CAD build for the part. Positions are in the model's coordinates, mm. A direction names the side the tool comes from. Coordinates: 2 decimals unless noted, no trailing zeros.
1) Wall check: line 1 along X through (y, z) = (-19, 4.5); line 2 along X through (y, z) = (-25.5, 2); line 3 along Y through (x, z) = (-2, 4.5). Give the ranges that are in metal, low to high.
2) Pin check, flat tips, straight feed: pin 1 Ø6 at (x, y) = (31.5, 18.5) entering from -Z; pin 2 Ø1.5 at (y, z) = (9.5, 3.5) entering from +X; pin 3 Ø6.5 at (y, z) = (-28, 5.5) entering from -X; pin 4 Ø5 at (y, z) = (15.5, 0.5) entering from +X. Stop position of each tip, or through.
3) Two-plate mould, pull along Y, no slides. Class faces 1 (the flat face through (13, -13, 0)), 2 (the cylindrical face through (-7, 6, 0)), 3 (the flat face through (22.815, 2.59, 2.465)), 4 (the flat face through (25, -50, 6)): +Y half, -Y half, draft (parallel to the pull), parting line (faces both ways), or undercut.
4) Which spindle directions (+Z, -Z, +X, -X, +Y, -Y) get a long thin tool onto all of the face, cutting with end or side? Do faces 5 (the flat face through (45, -22, 8)), 6 (the cylindrical face through (48, -22, 12)), 7 (the flat face through (-22, 0, -1)), 8 (the flat face through (22.81, -15.74, 2.46)), 9 (the flat face through (6, -6, 5)). Say none if no direction does.
5) Saw through at A-A, the plane y = -23. Give the number of separate pieces and of enclosed holes in the cut face, and give its area (3 significant figures).
```python
from build123d import *

# Parameters (mm, degrees)
F1_DEPTH  = 5
F3_DEPTH  = 5
F5_DEPTH  = 8
F6_SIZE   = 4.99999
F7_R      = 4.99999
F9_DEPTH  = 5
F11_DEPTH = 5


# Not quite as in the source:
# - a fillet or chamfer is up to 0.001 mm smaller than in the source, because OpenCascade refuses the exact size


with BuildPart() as f1:
    # F0 (on Top) → F1 (new body)
    with BuildSketch(Plane.XY):
        Polygon((0, 45), (-5, 45), (-5, 5), (-45, 5), (-45, 0), (0, -45), (0, -50), (50, -50), (50, 0), (45, 0), align=None)
        Polygon((45, -7.0710678119), (45, -45), (7.0710678119, -45), (-37.9289321881, 0), (0, 0), (0, 37.9289321881), align=None, mode=Mode.SUBTRACT)
    extrude(amount=F1_DEPTH)

    # F2 (on face) → F3 (join)
    with BuildSketch(Plane(origin=(0, 0, 0), x_dir=(1, 0, 0), z_dir=(0, 0, -1))):
        Polygon((0, -45), (0, 0), (-45, 0), (-45, -5), (-5, -5), (-5, -45), align=None)
    extrude(amount=F3_DEPTH)

    # F4 (on face) → F5 (join)
    with BuildSketch(Plane.XY.offset(5)):
        Polygon((50, 0), (45, 0), (45, -45), (0, -45), (0, -50), (50, -50), align=None)
    extrude(amount=F5_DEPTH)

    # F6 (size 5 in the source; OpenCascade refuses exactly that, so slightly less here)
    f6_edges = [f1.edges().sort_by_distance(p)[0] for p in [
        (0, -50, 6.5),
        (50, 0, 6.5),
    ]]
    chamfer(f6_edges, length=F6_SIZE)

    # F7 (radius 5 in the source; OpenCascade refuses exactly that, so slightly less here)
    f7_edges = [f1.edges().sort_by_distance(p)[0] for p in [
        (50, -50, 6.5),
        (-5, 45, 0),
        (-45, 5, 0),
        (-5, 5, 0),
        (50, -27.499995, 13),
        (27.499995, -50, 13),
        (27.499995, -50, 0),
        (50, -27.499995, 0),
    ]]
    fillet(f7_edges, radius=F7_R)

    # F8 (on Top) → F9 (join)
    with BuildSketch(Plane.XY):
        Polygon((0, 0), (-7.0710678119, 0), (37.9289321881, -45), (45, -45), (45, -37.9289321881), (0, 7.0710678119), align=None)
    extrude(amount=F9_DEPTH)

    # F10 (on Top) → F11 (join)
    with BuildSketch(Plane.XY):
        Polygon((45, -7.0710678119), (0, 12.524562237), (0, 7.0710678119), (45, -12.524562237), align=None)
        Polygon((12.524562237, -45), (-7.0710678119, 0), (-12.524562237, 0), (7.0710678119, -45), align=None)
    extrude(amount=F11_DEPTH)


solid = f1.part
```
Data:
1. line 1: x = -26 to -18.93, -4.25 to 1.2, 11.93 to 26.07, 45 to 49.97
1. line 2: x = -19.5 to -12.43, -1.42 to 4.03, 18.43 to 32.57, 45 to 49
1. line 3: y = -43 to -35.93, -24.17 to -11.65, -5.07 to 44.58
2. pin 1: passes through
2. pin 2: stops at x = 36.25
2. pin 3: stops at x = -20.21
2. pin 4: stops at x = 32
3. face 1: draft
3. face 2: +Y half
3. face 3: undercut
3. face 4: -Y half
4. face 5: +Z
4. face 6: +Z, +X, +Y, -Y
4. face 7: -Z
4. face 8: +Z, -Z
4. face 9: +Z, -X, +Y
5. separate pieces: 4
5. enclosed holes: 0
5. area: 188 mm2
